```python
from build123d import *

# Parameters (mm, degrees)
SKETCH1_W           = 5.08
SKETCH1_H           = 2.54
BOSS_EXTRUDE1_DEPTH = 33.02


with BuildPart() as part:
    # Sketch1 → Boss-Extrude1 (new body)
    with BuildSketch(Plane.XY):
        Polygon((-2.742413779, 4.75), (-5.484827557, 0), (-2.742413779, -4.75), (2.742413779, -4.75), (5.484827557, 0), (2.742413779, 4.75), align=None)
        Rectangle(SKETCH1_W, SKETCH1_H, mode=Mode.SUBTRACT)
    extrude(amount=BOSS_EXTRUDE1_DEPTH)


solid = part.part
```
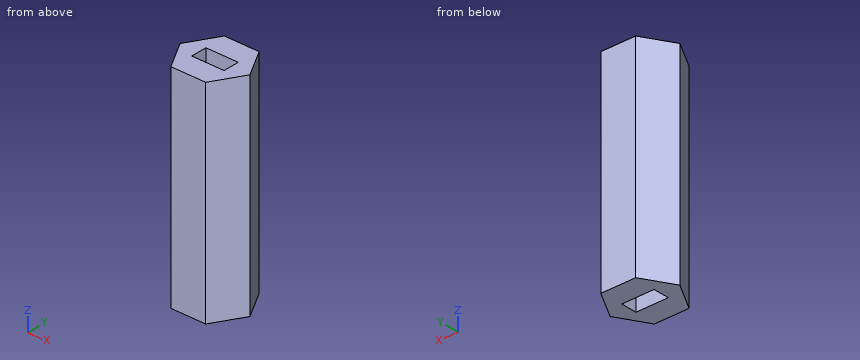
Could you check a few things on this model? Use its own coordinates, in mm. Coordinates: 2 decimals unless noted, no trailing zeros. Write each loop counter-clockwise with the first axis right and the second up, starting at its lowest first coordinate (ties: lowest second). Pieces come first, ordered by that corner, then holes. Notation, with made-up numbers: (-4.75, 11) -> (35.25, 11) arc R20 cw to (35.25, 18) -> close; hole circle Ø11 at (49, 20.25). An arc over 180 degrees is marked (long way). Write item = value, one per line. Start each with the question number.
(1) I want a section at A-A (x = -1). Please give me the cut outline in (y, z), plus the area to 3 significant figures.
(2) I need wall thicknesses on line 1 (Y direction, x = -0.5, z = 5); line 2 (X direction, y = 0.5, z = 12.5); line 3 (X direction, y = 1.5, z = 9.5). Which ranges of each line are inside material? Lowest first, please. Write a range as [from, to].
(3) I want a section at B-B (z = 15.5). Please give me the cut outline in (x, y), plus the area to 3 significant figures.
(4) I want a section at C-C (y = -0.75). Please give me the cut outline in (x, z).
(5) I want a section at D-D (y = 2.25). Please give me the cut outline in (x, z).
Result set:
q1.outline = (-4.75, 0) -> (-1.27, 0) -> (-1.27, 33.02) -> (-4.75, 33.02) -> close; (1.27, 0) -> (4.75, 0) -> (4.75, 33.02) -> (1.27, 33.02) -> close
q1.area = 230 mm2
q2.line_1 = [-4.75, -1.27], [1.27, 4.75]
q2.line_2 = [-5.2, -2.54], [2.54, 5.2]
q2.line_3 = [-4.62, 4.62]
q3.outline = (-5.48, 0) -> (-2.74, -4.75) -> (2.74, -4.75) -> (5.48, 0) -> (2.74, 4.75) -> (-2.74, 4.75) -> close; hole (-2.54, -1.27) -> (2.54, -1.27) -> (2.54, 1.27) -> (-2.54, 1.27) -> close
q3.area = 65.3 mm2
q4.outline = (-5.05, 0) -> (-2.54, 0) -> (-2.54, 33.02) -> (-5.05, 33.02) -> close; (2.54, 0) -> (5.05, 0) -> (5.05, 33.02) -> (2.54, 33.02) -> close
q5.outline = (-4.19, 0) -> (4.19, 0) -> (4.19, 33.02) -> (-4.19, 33.02) -> close
